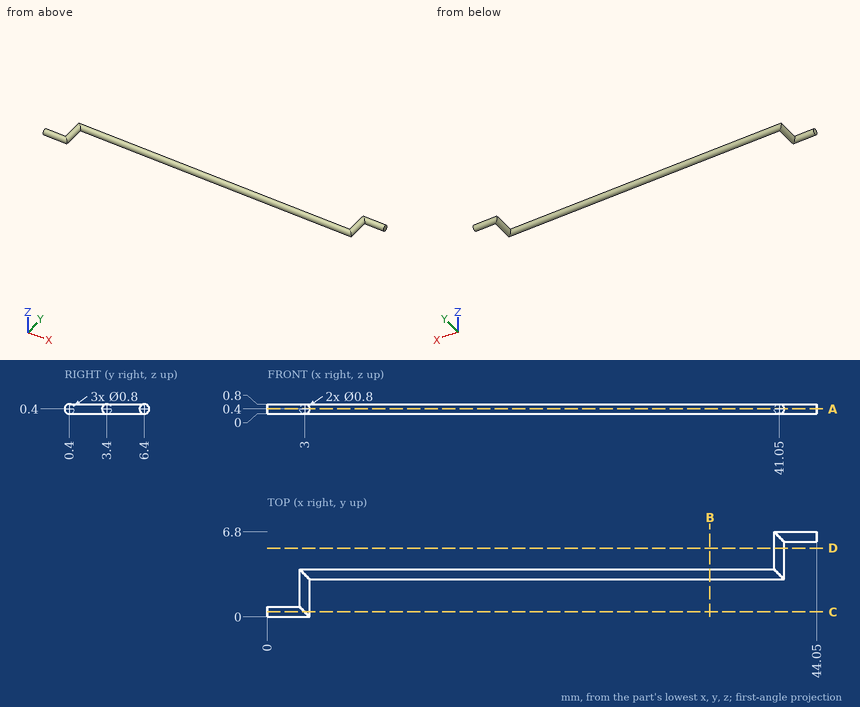
Answer from the drawing. Dimensions are ordinates in mm from the lowest x, y and z of the part. Round coordinates to 2 decimals unless told otherwise and drop trailing zeros. Loops run counter-clockwise (first coordinate to the right, second up) from the corner with the lowest first, then second, coordinate; pieces in that order, holes last. Notation, with made-up numbers: M 33.5,6.5 L 51.5,6.5 A35 cw 51.5,40.5 Z; hole C 73,62.25 d3. An arc over 180 degrees is marked long. One line per question, with ' | ' between items. Start each with the question number.
(1) A cutting plane is placed at A-A on z = 0.4. Write down the section's boundary in (x, y), plus the area to 3 significant figures.
(2) Find the intervals of material crossed by line 1 (Y direction, x = 9, z = 0.45); line 2 (X direction, y = 5.75, z = 0.4); line 3 (X direction, y = 1.75, z = 0.5), in increasing order.
(3) A cutting plane is placed at D-D on y = 5.5. Write down the section's boundary in (x, z), plus the area to 3 significant figures.
(4) A cutting plane is placed at C-C on y = 0.4. Write down the section's boundary in (x, z), plus the area to 3 significant figures.
(5) A cutting plane is placed at B-B on x = 35.5. Write down the section's boundary in (y, z).
Geometry check:
1) outline: M 0,0 L 3.4,0 L 3.4,3 L 41.45,3 L 41.45,6 L 44.05,6 L 44.05,6.8 L 40.65,6.8 L 40.65,3.8 L 2.6,3.8 L 2.6,0.8 L 0,0.8 Z | area: 40.0 mm²
2) line 1: y = 3 to 3.8 | line 2: x = 40.65 to 41.45 | line 3: x = 2.61 to 3.39
3) outline: C 41.05,0.4 d0.8 | area: 0.503 mm²
4) outline: M 0,0 L 3,0 A0.4 ccw 3,0.8 L 0,0.8 Z | area: 2.65 mm²
5) outline: C 3.4,0.4 d0.8
